```python
from build123d import *

# Parameters (mm, degrees)
SKETCH1_R           = 2.5
SKETCH1_R_2         = 22.5
SKETCH1_R_3         = 2
SKETCH1_R_4         = 6.5
SKETCH1_R_5         = 1.5
BOSS_EXTRUDE1_DEPTH = 5


with BuildPart() as part:
    # Sketch1 → Boss-Extrude1 (new body)
    with BuildSketch(Plane.XY):
        with BuildLine():
            Line((30.000692042, 92.545526446), (235.000692042, 92.545526446))
            ThreePointArc((235.000692042, 92.545526446), (238.536225947, 91.081060352), (240.000692042, 87.545526446))
            Line((240.000692042, 87.545526446), (240.000692042, -52.454473554))
            ThreePointArc((240.000692042, -52.454473554), (238.536225947, -55.99000746), (235.000692042, -57.454473554))
            Line((235.000692042, -57.454473554), (30.000692042, -57.454473554))
            ThreePointArc((30.000692042, -57.454473554), (-44.999307958, 17.545526446), (30.000692042, 92.545526446))
        make_face()
        with Locations((-34.999307958, 17.545526446)):
            Circle(SKETCH1_R, mode=Mode.SUBTRACT)
        with Locations((30.000692042, -47.454473554)):
            Circle(SKETCH1_R, mode=Mode.SUBTRACT)
        with Locations((30.000692042, 82.545526446)):
            Circle(SKETCH1_R, mode=Mode.SUBTRACT)
        with Locations((230.000692042, -47.454473554)):
            Circle(SKETCH1_R, mode=Mode.SUBTRACT)
        with Locations((230.000692042, 82.545526446)):
            Circle(SKETCH1_R, mode=Mode.SUBTRACT)
        with Locations((130.000692042, 82.545526446)):
            Circle(SKETCH1_R, mode=Mode.SUBTRACT)
        with Locations((130.000692042, -47.454473554)):
            Circle(SKETCH1_R, mode=Mode.SUBTRACT)
        with Locations((30.000692042, 17.545526446)):
            Circle(SKETCH1_R_2, mode=Mode.SUBTRACT)
        with Locations((61.815692042, 49.360526446)):
            Circle(SKETCH1_R_3, mode=Mode.SUBTRACT)
        with Locations((61.815692042, -14.269473554)):
            Circle(SKETCH1_R_3, mode=Mode.SUBTRACT)
        with Locations((-1.814307958, -14.269473554)):
            Circle(SKETCH1_R_3, mode=Mode.SUBTRACT)
        with Locations((-1.814307958, 49.360526446)):
            Circle(SKETCH1_R_3, mode=Mode.SUBTRACT)
        with Locations((192.000692042, 17.545526446)):
            Circle(SKETCH1_R_4, mode=Mode.SUBTRACT)
        with Locations((199.000692042, 33.045526446)):
            Circle(SKETCH1_R_5, mode=Mode.SUBTRACT)
        with Locations((199.000692042, 2.045526446)):
            Circle(SKETCH1_R_5, mode=Mode.SUBTRACT)
        with Locations((185.893407347, 25.818922843)):
            Circle(SKETCH1_R_5, mode=Mode.SUBTRACT)
        with Locations((212.107976736, 25.818922843)):
            Circle(SKETCH1_R_5, mode=Mode.SUBTRACT)
        with Locations((212.107976736, 9.272130049)):
            Circle(SKETCH1_R_5, mode=Mode.SUBTRACT)
        with Locations((185.893407347, 9.272130049)):
            Circle(SKETCH1_R_5, mode=Mode.SUBTRACT)
    extrude(amount=BOSS_EXTRUDE1_DEPTH)


solid = part.part
```
Verification items for the finished model (mm, model axes). Round coordinates to 2 decimals unless told otherwise and drop trailing zeros. Order: outer loops, then holes, each group sorted by start corner. A loop starts at its lowest first (then second) coordinate and runs counter-clockwise, first axis right, second up.
1) Draft check along Y on faces 1 (the flat face through (99, 19, 5)), 2 (the cylindrical face through (229.459, 80.105, 2.465)), 3 (the flat face through (134, -57.454, 2)). Enter one of: +Y half, -Y half, draft (parallel to the pull), parting line (faces both ways), or undercut.
Geometry says:
face 1: draft
face 2: undercut
face 3: -Y half
2) Cross-section at B-B, the plane x = -17.5. Record the cut outline in (y, z), plus the area to 3 significant figures.
Geometry says:
outline: (-40.49, 0) - (75.59, 0) - (75.59, 5) - (-40.49, 5) - close
area: 580 mm2
3) Cross-section at A-A, the plane z = 2.45. Give the number of separate pieces and of enclosed holes in the cut face, plus the area to 3 significant figures.
Geometry says:
separate pieces: 1
enclosed holes: 19
area: 38,400 mm2
4) Cross-section at C-C, the plane y = -25. Record the cut outline in (x, z), plus the area to 3 significant figures.
Geometry says:
outline: (-31.76, 0) - (240, 0) - (240, 5) - (-31.76, 5) - close
area: 1,360 mm2
5) Depth check by flat-ended pin: pin 1 (4 mm diameter, centred on x = 199, y = 2.05, fed in from +Z); pin 2 (1 mm diameter, centred on y = 63.5, z = 4.5, fed in from -X). Enter the tip coordinate at first touch or a pass-through.
Geometry says:
pin 1: stops at z = 5
pin 2: stops at x = -29.66
6) Material ranges on line 1 (Y direction, x = 213, z = 2.1); line 2 (X direction, y = 9.5, z = 4); line 3 (X direction, y = 10.5, z = 4.7) (3 decimals), recorded low to high.
Geometry says:
line 1: y = -57.45 to 8.07, 10.48 to 24.61, 27.02 to 92.55
line 2: x = -44.57 to 8.99, 51.01 to 184.41, 187.38 to 210.63, 213.59 to 240
line 3: x = -44.668 to 8.632, 51.369 to 185.032, 186.755 to 211.246, 212.97 to 240.001
